For this review, take the finished solid that the model builds, in its own axes (mm). Round coordinates to 2 decimals unless told otherwise and drop trailing zeros. Write each loop counter-clockwise with the first axis right and the second up, starting at its lowest first coordinate (ties: lowest second). Pieces come first, ordered by that corner, then holes.
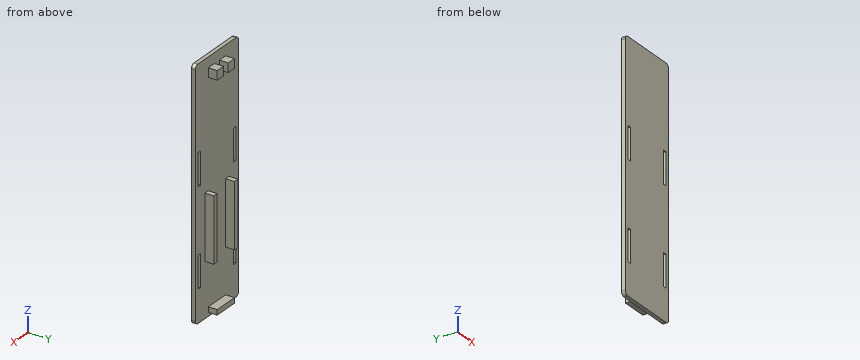
from build123d import *

# Parameters (mm, degrees)
SKETCH1_W           = 50
SKETCH1_H           = 190
BOSS_EXTRUDE1_DEPTH = 3
FILLET1_R           = 3
SKETCH2_W           = 20
SKETCH2_H           = 4
SKETCH2_W_2         = 4
SKETCH2_H_2         = 50
BOSS_EXTRUDE2_DEPTH = 7
SKETCH3_W           = 20
SKETCH3_H           = 7
BOSS_EXTRUDE3_DEPTH = 7
CUT_EXTRUDE1_DEPTH  = 7
SKETCH6_W           = 3
SKETCH6_H           = 25
CUT_EXTRUDE2_DEPTH  = 7


with BuildPart() as part:
    # Sketch1 → Boss-Extrude1 (new body)
    with BuildSketch(Plane(origin=(0, 0, 0), x_dir=(1, 0, 0), z_dir=(0, 1, 0))):
        with Locations((25, 95)):
            Rectangle(SKETCH1_W, SKETCH1_H)
    extrude(amount=BOSS_EXTRUDE1_DEPTH)

    # Fillet1
    fillet1_edges = [part.edges().sort_by_distance(p)[0] for p in [
        (0, 1.5, -190),
        (50, 1.5, -190),
        (50, 1.5, 0),
        (0, 1.5, 0),
    ]]
    fillet(fillet1_edges, radius=FILLET1_R)

    # Sketch2 → Boss-Extrude2 (add)
    with BuildSketch(Plane(origin=(0, 3, 0), x_dir=(1, 0, 0), z_dir=(0, 1, 0))):
        with Locations((25, 185)):
            Rectangle(SKETCH2_W, SKETCH2_H)
        with Locations((13, 123)):
            Rectangle(SKETCH2_W_2, SKETCH2_H_2)
        with Locations((37, 123)):
            Rectangle(SKETCH2_W_2, SKETCH2_H_2)
    extrude(amount=BOSS_EXTRUDE2_DEPTH)

    # Sketch3 → Boss-Extrude3 (add)
    with BuildSketch(Plane(origin=(0, 3, 0), x_dir=(1, 0, 0), z_dir=(0, 1, 0))):
        with Locations((25, 11.5)):
            Rectangle(SKETCH3_W, SKETCH3_H)
    extrude(amount=BOSS_EXTRUDE3_DEPTH)

    # Sketch5 → Cut-Extrude1 (cut)
    with BuildSketch(Plane(origin=(0, 0, -15), x_dir=(-1, 0, 0), z_dir=(0, 0, -1))):
        Polygon((-22.15, 3), (-22.35, 10), (-27.65, 10), (-27.85, 3), align=None)
    extrude(amount=-CUT_EXTRUDE1_DEPTH, mode=Mode.SUBTRACT)

    # Sketch6 → Cut-Extrude2 (cut)
    with BuildSketch(Plane(origin=(0, 3, 0), x_dir=(1, 0, 0), z_dir=(0, 1, 0))):
        with Locations((4.5, 152.5)):
            Rectangle(SKETCH6_W, SKETCH6_H)
        with Locations((45.5, 152.5)):
            Rectangle(SKETCH6_W, SKETCH6_H)
        with Locations((4.5, 77.5)):
            Rectangle(SKETCH6_W, SKETCH6_H)
        with Locations((45.5, 77.5)):
            Rectangle(SKETCH6_W, SKETCH6_H)
    extrude(amount=-CUT_EXTRUDE2_DEPTH, mode=Mode.SUBTRACT)


solid = part.part
(1) We need section B-B, the plane x = 30. Give the boundary of the cut face in (y, z), and give its area (3 significant figures).
Geometry check:
outline: (0, -190) - (3, -190) - (3, -187) - (10, -187) - (10, -183) - (3, -183) - (3, -15) - (10, -15) - (10, -8) - (3, -8) - (3, 0) - (0, 0) - close
area: 647 mm2
(2) We need section C-C, the plane y = 8.5. Give the boundary of the cut face in (x, z), and give its area (3 significant figures).
Geometry check:
outline: (11, -148) - (15, -148) - (15, -98) - (11, -98) - close; (15, -187) - (35, -187) - (35, -183) - (15, -183) - close; (15, -15) - (22.31, -15) - (22.31, -8) - (15, -8) - close; (27.69, -15) - (35, -15) - (35, -8) - (27.69, -8) - close; (35, -148) - (39, -148) - (39, -98) - (35, -98) - close
area: 582 mm2
(3) We need section A-A, the plane z = -70.5. Give the boundary of the cut face in (x, y).
Geometry check:
outline: (0, 0) - (3, 0) - (3, 3) - (0, 3) - close; (6, 0) - (44, 0) - (44, 3) - (6, 3) - close; (47, 0) - (50, 0) - (50, 3) - (47, 3) - close
(4) For line 1 along Z through (x, y) = (20, 6); line 2 along X through (y, z) = (7, -131); line 3 along Z through (x, y) = (46.5, 0.5), list the stretches that pass through material, from the lowest coordinate up.
Geometry check:
line 1: z = -187 to -183, -15 to -8
line 2: x = 11 to 15, 35 to 39
line 3: z = -190 to -165, -140 to -90, -65 to 0
(5) For pin 1 Ø2 at (y, z) = (7, -185.5) entering from -X; pin 2 Ø2 at (y, z) = (7.5, -127.5) entering from +X; pin 3 Ø3 at (y, z) = (6.5, -126) entering from -X, all flat-tipped, find the tip position at first contact; note any pin that passes through.
Geometry check:
pin 1: stops at x = 15
pin 2: stops at x = 39
pin 3: stops at x = 11
(6) We need section D-D, the plane z = -114.5. Give the boundary of the cut face in (x, y), and give its area (3 significant figures).
Geometry check:
outline: (0, 0) - (50, 0) - (50, 3) - (39, 3) - (39, 10) - (35, 10) - (35, 3) - (15, 3) - (15, 10) - (11, 10) - (11, 3) - (0, 3) - close
area: 206 mm2
